```python
from build123d import *

# Parameters (mm, degrees)
F1_DEPTH = 25
F3_DEPTH = 37.5
F5_DEPTH = 5


with BuildPart() as f1:
    # F0 (on Front) → F1 (new body)
    with BuildSketch(Plane.XZ):
        with BuildLine():
            Line((205, 150), (-205, 150))
            ThreePointArc((-205, 150), (-219.142136, 144.142136), (-225, 130))
            Line((-225, 130), (-225, -130))
            ThreePointArc((-225, -130), (-219.142136, -144.142136), (-205, -150))
            Line((-205, -150), (205, -150))
            ThreePointArc((205, -150), (219.142136, -144.142136), (225, -130))
            Line((225, -130), (225, 130))
            ThreePointArc((225, 130), (219.142136, 144.142136), (205, 150))
        make_face()
    extrude(amount=F1_DEPTH)

    # F2 (on Right) → F3 (join, symmetric)
    with BuildSketch(Plane.YZ):
        with BuildLine():
            Line((60, -200), (21.404476, -6.935301))
            ThreePointArc((21.404476, -6.935301), (-15.255166, 16.53874), (5.187273, -21.893885))
            Line((5.187273, -21.893885), (30, -200))
            Line((30, -200), (60, -200))
        make_face()
    extrude(amount=F3_DEPTH, both=True)

    # F4 (on face) → F5 (join)
    with BuildSketch(Plane(origin=(0, 0, -200), x_dir=(1, 0, 0), z_dir=(0, 0, -1))):
        with BuildLine():
            Line((92.5, 70), (-92.5, 70))
            ThreePointArc((-92.5, 70), (-106.642136, 64.142136), (-112.5, 50))
            Line((-112.5, 50), (-112.5, -90))
            ThreePointArc((-112.5, -90), (-106.642136, -104.142136), (-92.5, -110))
            Line((-92.5, -110), (92.5, -110))
            ThreePointArc((92.5, -110), (106.642136, -104.142136), (112.5, -90))
            Line((112.5, -90), (112.5, 50))
            ThreePointArc((112.5, 50), (106.642136, 64.142136), (92.5, 70))
        make_face()
    extrude(amount=F5_DEPTH)


solid = f1.part
```
Read the model definition and answer for the solid it produces. Units are mm, in the model's axes. A direction names the side the tool comes from. Give positions to 0.01 mm unless a question says otherwise; leave off trailing zeros. Order: outer loops, then holes, each group sorted by start corner. A loop starts at its lowest first (then second) coordinate and runs counter-clockwise, first axis right, second up.
(1) For a pull along Z with two mould halves and no side action, classify faces 1 (the flat face through (-2, 19, -205)), 2 (the cylindrical face through (219.297, -12.325, 143.986)), 3 (the cylindrical face through (0.52, 18.37, 12.99)) as released by +Z, released by -Z, zero draft, split by the parting line, or undercut.
(2) Straight lines are drawn through the part: L1, parallel to Z at x = 75.5, y = -15; L2, parallel to Y at x = -60, z = 61; L3, parallel to Z at x = -105.5, y = 15.5. For each, find the intervals that lie inside material, in ascending order.
(3) For faces 4 (the flat face through (37.5, 30, -87)), 5 (the flat face through (-37.5, 30, -87)), 6 (the flat face through (-3, -25, 2)), determine the directions among +Z, -Z, +X, -X, +Y, -Y from which every point of the face is accessible in a straight line to the end or side of a thin tool.
(4) Find section A-A (x = 61). Give the vertices of the cut face in (y, z).
(5) Find section B-B (z = -76). Give the vertices of the cut face in (x, y).
(6) Find section C-C (y = 52.5). Give the vertices of the cut face in (x, z).
(7) Find section D-D (x = 122). Give the vertices of the cut face in (y, z), plus the area to 3 significant figures.
(8) Given pin 1 (1 mm diameter, centred on x = -76, y = 39, fed in from +Z); pin 2 (5.5 mm diameter, centred on y = -5.5, z = -202, fed in from -X); pin 3 (1.5 mm diameter, centred on y = 26, z = -203, fed in from +X), each flat-ended and moving along its own axis, determine where each tip first touches the part or whether it passes through.
Result sheet:
1. face 1: released by -Z
1. face 2: released by +Z
1. face 3: undercut
2. L1: z = -205 to -200, -150 to 150
2. L2: y = -25 to 0
2. L3: z = -205 to -200
3. face 4: +Z, +X, +Y
3. face 5: +Z, -X, +Y
3. face 6: +Z, +X, -X, -Y
4. outline: (-70, -205) - (110, -205) - (110, -200) - (-70, -200) - close; (-25, -150) - (0, -150) - (0, 150) - (-25, 150) - close
5. outline: (-225, -25) - (225, -25) - (225, 0) - (-225, 0) - close; (-37.5, 12.73) - (37.5, 12.73) - (37.5, 35.21) - (-37.5, 35.21) - close
6. outline: (-112.5, -205) - (112.5, -205) - (112.5, -200) - (37.5, -200) - (37.5, -162.48) - (-37.5, -162.48) - (-37.5, -200) - (-112.5, -200) - close
7. outline: (-25, -150) - (0, -150) - (0, 150) - (-25, 150) - close
7. area: 7,500 mm2
8. pin 1: stops at z = -200
8. pin 2: stops at x = -112.5
8. pin 3: stops at x = 112.5
